Read the model definition and answer for the solid it produces. Units are mm, in the model's axes. A direction names the side the tool comes from. Give positions to 0.01 mm unless a question says otherwise; leave off trailing zeros. Write each loop counter-clockwise with the first axis right and the second up, starting at its lowest first coordinate (ties: lowest second). Pieces come first, ordered by that corner, then holes.
```python
from build123d import *

# Parameters (mm, degrees)
F0_W     = 180
F0_H     = 30.7765754297
F1_DEPTH = 2


with BuildPart() as f1:
    # F0 (on Front) → F1 (new body)
    with BuildSketch(Plane.XZ):
        with Locations((37.3380143768, 10.3882877148)):
            Rectangle(F0_W, F0_H)
        with BuildLine():
            add(Edge.make_bspline(
                [(-29.3945604163, 8.9251803522), (-28.1343492982, 7.6920220666), (-28.1343492982, 5.6630596223)],
                knots=[0, 0, 0, 1, 1, 1], degree=2))
            add(Edge.make_bspline(
                [(-28.1343492982, 5.6630596223), (-28.1343492982, 2.9577763633), (-30.1633117425, 1.4788881816)],
                knots=[0, 0, 0, 1, 1, 1], degree=2))
            add(Edge.make_bspline(
                [(-30.1633117425, 1.4788881816), (-32.1922741868, 0), (-35.7993185322, 0)],
                knots=[0, 0, 0, 1, 1, 1], degree=2))
            Line((-35.7993185322, 0), (-45.7322168984, 0))
            Line((-45.7322168984, 0), (-45.7322168984, 19.8522703161))
            Line((-45.7322168984, 19.8522703161), (-36.6424651479, 19.8522703161))
            add(Edge.make_bspline(
                [(-36.6424651479, 19.8522703161), (-33.0083679699, 19.8522703161), (-31.1417225212, 18.592059198)],
                knots=[0, 0, 0, 1, 1, 1], degree=2))
            add(Edge.make_bspline(
                [(-31.1417225212, 18.592059198), (-29.2750770724, 17.3318480798), (-29.2750770724, 14.8655315086)],
                knots=[0, 0, 0, 1, 1, 1], degree=2))
            add(Edge.make_bspline(
                [(-29.2750770724, 14.8655315086), (-29.2750770724, 13.1747294717), (-30.2106541995, 12.0114576703)],
                knots=[0, 0, 0, 1, 1, 1], degree=2))
            add(Edge.make_bspline(
                [(-30.2106541995, 12.0114576703), (-31.1462313266, 10.8481858689), (-33.0624736351, 10.44239338)],
                knots=[0, 0, 0, 1, 1, 1], degree=2))
            add(Edge.make_bspline(
                [(-33.0624736351, 10.44239338), (-30.6547715345, 10.1583386378), (-29.3945604163, 8.9251803522)],
                knots=[0, 0, 0, 1, 1, 1], degree=2))
        make_face(mode=Mode.SUBTRACT)
        Polygon((-10.0810923493, 0), (-24.8925181927, 0), (-24.8925181927, 19.8522703161), (-20.7353995846, 19.8522703161), (-20.7353995846, 3.2147782729), (-10.0810923493, 3.2147782729), align=None, mode=Mode.SUBTRACT)
        Polygon((10.8803441031, 0), (6.7683135493, 0), (5.0053706255, 5.0724061108), (-2.5604048891, 5.0724061108), (-4.3233478129, 0), (-8.480466421, 0), (-1.2348160921, 19.8522703161), (3.6662554122, 19.8522703161), align=None, mode=Mode.SUBTRACT)
        with BuildLine():
            add(Edge.make_bspline(
                [(18.5114972964, 4.792860174), (20.0106751024, 2.9893380013), (22.8422049136, 2.9893380013)],
                knots=[0, 0, 0, 1, 1, 1], degree=2))
            add(Edge.make_bspline(
                [(22.8422049136, 2.9893380013), (26.6070574491, 2.9893380013), (28.0724192145, 6.7632081477)],
                knots=[0, 0, 0, 1, 1, 1], degree=2))
            Line((28.0724192145, 6.7632081477), (31.6929899762, 5.3970401018))
            add(Edge.make_bspline(
                [(31.6929899762, 5.3970401018), (30.5252093694, 2.5204222364), (28.2617890426, 1.1181837471)],
                knots=[0, 0, 0, 1, 1, 1], degree=2))
            add(Edge.make_bspline(
                [(28.2617890426, 1.1181837471), (25.9983687158, -0.2840547422), (22.8422049136, -0.2840547422)],
                knots=[0, 0, 0, 1, 1, 1], degree=2))
            add(Edge.make_bspline(
                [(22.8422049136, -0.2840547422), (18.053853545, -0.2840547422), (15.4410007973, 2.4302461277)],
                knots=[0, 0, 0, 1, 1, 1], degree=2))
            add(Edge.make_bspline(
                [(15.4410007973, 2.4302461277), (12.8281480496, 5.1445469977), (12.8281480496, 10.0185656694)],
                knots=[0, 0, 0, 1, 1, 1], degree=2))
            add(Edge.make_bspline(
                [(12.8281480496, 10.0185656694), (12.8281480496, 14.9061107575), (15.348570286, 17.5279811161)],
                knots=[0, 0, 0, 1, 1, 1], degree=2))
            add(Edge.make_bspline(
                [(15.348570286, 17.5279811161), (17.8689925223, 20.1498514746), (22.6618526963, 20.1498514746)],
                knots=[0, 0, 0, 1, 1, 1], degree=2))
            add(Edge.make_bspline(
                [(22.6618526963, 20.1498514746), (26.156176906, 20.1498514746), (28.3542195539, 18.7476129854)],
                knots=[0, 0, 0, 1, 1, 1], degree=2))
            add(Edge.make_bspline(
                [(28.3542195539, 18.7476129854), (30.5522622019, 17.3453744961), (31.440496872, 14.6265648207)],
                knots=[0, 0, 0, 1, 1, 1], degree=2))
            Line((31.440496872, 14.6265648207), (27.774838056, 13.6256100149))
            add(Edge.make_bspline(
                [(27.774838056, 13.6256100149), (27.3104310965, 15.1180246128), (25.9510262588, 15.9994960747)],
                knots=[0, 0, 0, 1, 1, 1], degree=2))
            add(Edge.make_bspline(
                [(25.9510262588, 15.9994960747), (24.5916214211, 16.8809675366), (22.7475199995, 16.8809675366)],
                knots=[0, 0, 0, 1, 1, 1], degree=2))
            add(Edge.make_bspline(
                [(22.7475199995, 16.8809675366), (19.9295166047, 16.8809675366), (18.4709180475, 15.1338054318)],
                knots=[0, 0, 0, 1, 1, 1], degree=2))
            add(Edge.make_bspline(
                [(18.4709180475, 15.1338054318), (17.0123194903, 13.386643327), (17.0123194903, 10.0185656694)],
                knots=[0, 0, 0, 1, 1, 1], degree=2))
            add(Edge.make_bspline(
                [(17.0123194903, 10.0185656694), (17.0123194903, 6.5963823467), (18.5114972964, 4.792860174)],
                knots=[0, 0, 0, 1, 1, 1], degree=2))
        make_face(mode=Mode.SUBTRACT)
        Polygon((53.055710112, 0), (48.1501298022, 0), (41.0217084145, 9.1168045831), (38.5689182597, 7.2411415234), (38.5689182597, 0), (34.4117996515, 0), (34.4117996515, 19.8522703161), (38.5689182597, 19.8522703161), (38.5689182597, 10.8481858689), (47.5143882363, 19.8522703161), (52.3613540755, 19.8522703161), (43.8802910583, 11.4568746022), align=None, mode=Mode.SUBTRACT)
        with BuildLine():
            add(Edge.make_bspline(
                [(68.2075507655, 4.792860174), (69.7067285716, 2.9893380013), (72.5382583827, 2.9893380013)],
                knots=[0, 0, 0, 1, 1, 1], degree=2))
            add(Edge.make_bspline(
                [(72.5382583827, 2.9893380013), (76.3031109183, 2.9893380013), (77.7684726836, 6.7632081477)],
                knots=[0, 0, 0, 1, 1, 1], degree=2))
            Line((77.7684726836, 6.7632081477), (81.3890434453, 5.3970401018))
            add(Edge.make_bspline(
                [(81.3890434453, 5.3970401018), (80.2212628385, 2.5204222364), (77.9578425117, 1.1181837471)],
                knots=[0, 0, 0, 1, 1, 1], degree=2))
            add(Edge.make_bspline(
                [(77.9578425117, 1.1181837471), (75.694422185, -0.2840547422), (72.5382583827, -0.2840547422)],
                knots=[0, 0, 0, 1, 1, 1], degree=2))
            add(Edge.make_bspline(
                [(72.5382583827, -0.2840547422), (67.7499070142, -0.2840547422), (65.1370542664, 2.4302461277)],
                knots=[0, 0, 0, 1, 1, 1], degree=2))
            add(Edge.make_bspline(
                [(65.1370542664, 2.4302461277), (62.5242015187, 5.1445469977), (62.5242015187, 10.0185656694)],
                knots=[0, 0, 0, 1, 1, 1], degree=2))
            add(Edge.make_bspline(
                [(62.5242015187, 10.0185656694), (62.5242015187, 14.9061107575), (65.0446237551, 17.5279811161)],
                knots=[0, 0, 0, 1, 1, 1], degree=2))
            add(Edge.make_bspline(
                [(65.0446237551, 17.5279811161), (67.5650459915, 20.1498514746), (72.3579061654, 20.1498514746)],
                knots=[0, 0, 0, 1, 1, 1], degree=2))
            add(Edge.make_bspline(
                [(72.3579061654, 20.1498514746), (75.8522303751, 20.1498514746), (78.0502730231, 18.7476129854)],
                knots=[0, 0, 0, 1, 1, 1], degree=2))
            add(Edge.make_bspline(
                [(78.0502730231, 18.7476129854), (80.2483156711, 17.3453744961), (81.1365503411, 14.6265648207)],
                knots=[0, 0, 0, 1, 1, 1], degree=2))
            Line((81.1365503411, 14.6265648207), (77.4708915251, 13.6256100149))
            add(Edge.make_bspline(
                [(77.4708915251, 13.6256100149), (77.0064845656, 15.1180246128), (75.6470797279, 15.9994960747)],
                knots=[0, 0, 0, 1, 1, 1], degree=2))
            add(Edge.make_bspline(
                [(75.6470797279, 15.9994960747), (74.2876748903, 16.8809675366), (72.4435734687, 16.8809675366)],
                knots=[0, 0, 0, 1, 1, 1], degree=2))
            add(Edge.make_bspline(
                [(72.4435734687, 16.8809675366), (69.6255700738, 16.8809675366), (68.1669715166, 15.1338054318)],
                knots=[0, 0, 0, 1, 1, 1], degree=2))
            add(Edge.make_bspline(
                [(68.1669715166, 15.1338054318), (66.7083729594, 13.386643327), (66.7083729594, 10.0185656694)],
                knots=[0, 0, 0, 1, 1, 1], degree=2))
            add(Edge.make_bspline(
                [(66.7083729594, 10.0185656694), (66.7083729594, 6.5963823467), (68.2075507655, 4.792860174)],
                knots=[0, 0, 0, 1, 1, 1], degree=2))
        make_face(mode=Mode.SUBTRACT)
        Polygon((102.2557949836, 0), (98.1437644298, 0), (96.380821506, 5.0724061108), (88.8150459915, 5.0724061108), (87.0521030676, 0), (82.8949844595, 0), (90.1406347884, 19.8522703161), (95.0417062928, 19.8522703161), align=None, mode=Mode.SUBTRACT)
        Polygon((120.3361047651, 16.6420008487), (113.9110570248, 16.6420008487), (113.9110570248, 0), (109.7539384167, 0), (109.7539384167, 16.6420008487), (103.3424170927, 16.6420008487), (103.3424170927, 19.8522703161), (120.3361047651, 19.8522703161), align=None, mode=Mode.SUBTRACT)
    extrude(amount=F1_DEPTH)


solid = f1.part
```
Item 1: Find the intervals of material crossed by line 1 along Z through (x, y) = (-44, -1); line 2 along Z through (x, y) = (107, -0.8), in increasing order.
Result set:
line 1: z = -5 to 0, 19.85 to 25.78
line 2: z = -5 to 16.64, 19.85 to 25.78
Item 2: Which of the six approach directions +Z, -Z, +X, -X, +Y, -Y give full straight-line access (tool end or side, diameter ignored) to faces 1 (the flat face through (-4.908, -0.986, 9.787)), 2 (the flat face through (56, 0, 11))?
Result set:
face 1: +Y, -Y
face 2: +Z, -Z, +X, -X, +Y
Item 3: Section A-A (x = 105.5) is taken. Write down the section's boundary in (y, z).
Result set:
outline: (-2, -5) - (0, -5) - (0, 16.64) - (-2, 16.64) - close; (-2, 19.85) - (0, 19.85) - (0, 25.78) - (-2, 25.78) - close
Item 4: Section B-B (y = -1.3) is taken. Give the number of separate pieces and of enclosed holes in the cut face, and give its area (3 significant figures).
Result set:
separate pieces: 1
enclosed holes: 8
area: 4,080 mm2
Item 5: Determine the mould class of faces 3 (the flat face through (98.598, -0.986, 10.065)), 4 (the flat face through (56, -2, 11)) for opening direction Z: pulls with the +Z half, pulls with the -Z half, needs draft (parallel to the pull), parting line crosses it, or undercut.
Result set:
face 3: undercut
face 4: needs draft
